Build history of the part. All positions in model axes, mm. Face numbers are marked on the shaded views. A direction names the side the tool comes from. Round coordinates to 2 decimals unless told otherwise and drop trailing zeros. Write each loop counter-clockwise with the first axis right and the second up, starting at its lowest first coordinate (ties: lowest second). Pieces come first, ordered by that corner, then holes. Notation, with made-up numbers: (15.25, -23) -> (48.25, -23) arc R25 ccw to (48.25, -2) -> close; hole circle Ø8 at (7.5, 59). An arc over 180 degrees is marked (long way). Answer in a Markdown table with one row per item.
```python
from build123d import *

# Parameters (mm, degrees)
SKETCH1_W           = 168.045783506
SKETCH1_H           = 95.010377358
BOSS_EXTRUDE1_DEPTH = 5
SKETCH2_W           = 168.045783506
SKETCH2_H           = 95.010377358
SKETCH2_W_2         = 148.045783506
SKETCH2_H_2         = 75.010377358
BOSS_EXTRUDE2_DEPTH = 30
SKETCH3_W           = 15
SKETCH3_H           = 15
SKETCH3_W_2         = 43.208090913
SKETCH3_H_2         = 75.010377358
BOSS_EXTRUDE3_DEPTH = 5


with BuildPart() as part:
    # Sketch1 → Boss-Extrude1 (new body)
    with BuildSketch(Plane(origin=(0, 0, 0), x_dir=(1, 0, 0), z_dir=(0, 1, 0))):
        with Locations((84.022891753, 47.505188679)):
            Rectangle(SKETCH1_W, SKETCH1_H)
    extrude(amount=BOSS_EXTRUDE1_DEPTH)

    # Sketch2 → Boss-Extrude2 (add)
    with BuildSketch(Plane(origin=(0, 5, 0), x_dir=(1, 0, 0), z_dir=(0, 1, 0))):
        with Locations((84.022891753, 47.505188679)):
            Rectangle(SKETCH2_W, SKETCH2_H)
        with Locations((84.022891753, 47.505188679)):
            Rectangle(SKETCH2_W_2, SKETCH2_H_2, mode=Mode.SUBTRACT)
    extrude(amount=BOSS_EXTRUDE2_DEPTH)

    # Sketch3 → Boss-Extrude3 (add)
    with BuildSketch(Plane(origin=(0, 5, 0), x_dir=(1, 0, 0), z_dir=(0, 1, 0))):
        with Locations((17.5, 77.510377358)):
            Rectangle(SKETCH3_W, SKETCH3_H)
        with Locations((17.5, 17.5)):
            Rectangle(SKETCH3_W, SKETCH3_H)
        with Locations((136.44173805, 47.505188679)):
            Rectangle(SKETCH3_W_2, SKETCH3_H_2)
    extrude(amount=BOSS_EXTRUDE3_DEPTH)


solid = part.part
```
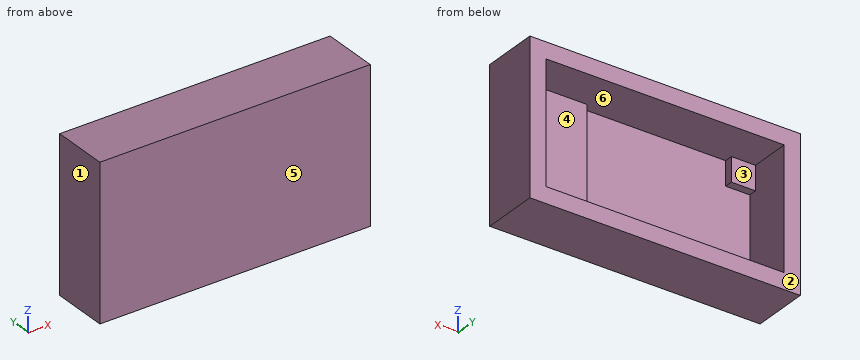
Q1. Wall check: line 1 (X direction, y = 28.5, z = -34.5); line 2 (Z direction, x = 112, y = 20); line 3 (X direction, y = 5.5, z = -49.5). Give the ranges that are in metal, low to high. Write a range as [from, to].
A:
| item | result |
|---|---|
| line 1 | [0, 10], [158.05, 168.05] |
| line 2 | [-95.01, -85.01], [-10, 0] |
| line 3 | [0, 10], [114.84, 168.05] |
Q2. Saw through at A-A on y = 23.5. Write the cut outline in (x, z).
A:
| item | result |
|---|---|
| outline | (0, -95.01) -> (168.05, -95.01) -> (168.05, 0) -> (0, 0) -> close; hole (10, -85.01) -> (158.05, -85.01) -> (158.05, -10) -> (10, -10) -> close |
Q3. Drop flat-ended pins along their axis: P1, Ø12, axis at x = 19.5, z = -74.5, coming from the +Y side; P2, Ø12, axis at x = 19, z = -15.5, coming from the +Y side. Give the stop position or say it passes through.
A:
| item | result |
|---|---|
| P1 | y = 10 |
| P2 | y = 35 |
Q4. Saw through at D-D on x = 41.5. Write the cut outline in (y, z).
A:
| item | result |
|---|---|
| outline | (0, -95.01) -> (35, -95.01) -> (35, -85.01) -> (5, -85.01) -> (5, -10) -> (35, -10) -> (35, 0) -> (0, 0) -> close |
Q5. Two-plate mould, pull along X, no slides. Class the marked faces 1, 2, 3 and 4: released by +X, released by -X, zero draft, split by the parting line, or undercut.
A:
| item | result |
|---|---|
| face 1 | released by -X |
| face 2 | zero draft |
| face 3 | undercut |
| face 4 | undercut |
Q6. Saw through at B-B on x = 128. Write the cut outline in (y, z), plus the area to 3 significant figures.
A:
| item | result |
|---|---|
| outline | (0, -95.01) -> (35, -95.01) -> (35, -85.01) -> (10, -85.01) -> (10, -10) -> (35, -10) -> (35, 0) -> (0, 0) -> close |
| area | 1,450 mm² |
Q7. Saw through at C-C on z = -47. Write the cut outline in (x, y).
A:
| item | result |
|---|---|
| outline | (0, 0) -> (168.05, 0) -> (168.05, 35) -> (158.05, 35) -> (158.05, 10) -> (114.84, 10) -> (114.84, 5) -> (10, 5) -> (10, 35) -> (0, 35) -> close |
Q8. Which spindle directions (+Z, -Z, +X, -X, +Y, -Y) get a long thin tool onto all of the face, cutting with end or side? Do the marked faces 5 and 6. Say none if no direction does.
A:
| item | result |
|---|---|
| face 5 | +Z, -Z, +X, -X, -Y |
| face 6 | +Y |
